For this review, take the finished solid that the model builds, in its own axes (mm). A direction names the side the tool comes from. Round coordinates to 2 decimals unless told otherwise and drop trailing zeros. Write each loop counter-clockwise with the first axis right and the second up, starting at its lowest first coordinate (ties: lowest second). Pieces come first, ordered by that corner, then holes.
from build123d import *

# Parameters (mm, degrees)
SKETCH1_R           = 2.032
BOSS_EXTRUDE1_DEPTH = 2.54
BOSS_EXTRUDE2_DEPTH = 7.62
SKETCH4_R           = 2.032
BOSS_EXTRUDE3_DEPTH = 2.54
CUT_EXTRUDE2_DEPTH  = 6.35
FILLET1_R           = 2.54
FILLET2_R           = 0.635
SKETCH6_R           = 1.95
CUT_EXTRUDE3_DEPTH  = 13.7


with BuildPart() as part:
    # Sketch1 → Boss-Extrude1 (new body)
    with BuildSketch(Plane(origin=(0, 0, 0), x_dir=(0, 0, -1), z_dir=(1, 0, 0))):
        with BuildLine():
            Line((19.05, 0), (0, 0))
            Line((0, 0), (-6.736031019, 0))
            ThreePointArc((-6.736031019, 0), (-5.127948142, 11.168903642), (-12.887784973, 19.361294713))
            Line((-12.887784973, 19.361294713), (-44.861814719, 46.190691279))
            ThreePointArc((-44.861814719, 46.190691279), (-45.74830741, 52.924271785), (-39.11761314, 54.394261314))
            Line((-39.11761314, 54.394261314), (15.875, 22.644261314))
            ThreePointArc((15.875, 22.644261314), (18.199261314, 20.32), (19.05, 17.145))
            Line((19.05, 17.145), (19.05, 0))
        make_face()
        with Locations((3.175, 6.35)):
            Circle(SKETCH1_R, mode=Mode.SUBTRACT)
        with Locations((15.875, 6.35)):
            Circle(SKETCH1_R, mode=Mode.SUBTRACT)
    extrude(amount=BOSS_EXTRUDE1_DEPTH)

    # Sketch1_4 → Boss-Extrude2 (add)
    with BuildSketch(Plane(origin=(0, 0, 0), x_dir=(0, 0, -1), z_dir=(1, 0, 0))):
        with BuildLine():
            Line((-6.736031019, 0), (0, 0))
            Line((0, 0), (0, 12.7))
            Line((0, 12.7), (19.05, 12.7))
            Line((19.05, 12.7), (19.05, 17.145))
            ThreePointArc((19.05, 17.145), (18.199261314, 20.32), (15.875, 22.644261314))
            Line((15.875, 22.644261314), (-39.11761314, 54.394261314))
            ThreePointArc((-39.11761314, 54.394261314), (-45.74830741, 52.924271785), (-44.861814719, 46.190691279))
            Line((-44.861814719, 46.190691279), (-12.887784973, 19.361294713))
            ThreePointArc((-12.887784973, 19.361294713), (-5.127948142, 11.168903642), (-6.736031019, 0))
        make_face()
    extrude(amount=-BOSS_EXTRUDE2_DEPTH)

    # Sketch4 → Boss-Extrude3 (add)
    with BuildSketch(Plane.ZY.offset(7.62)):
        with BuildLine():
            Line((-19.05, 0), (6.736031019, 0))
            ThreePointArc((6.736031019, 0), (5.127948142, 11.168903642), (12.887784973, 19.361294713))
            Line((12.887784973, 19.361294713), (44.861814719, 46.190691279))
            ThreePointArc((44.861814719, 46.190691279), (45.74830741, 52.924271785), (39.11761314, 54.394261314))
            Line((39.11761314, 54.394261314), (-15.875, 22.644261314))
            ThreePointArc((-15.875, 22.644261314), (-18.199261314, 20.32), (-19.05, 17.145))
            Line((-19.05, 17.145), (-19.05, 0))
        make_face()
        with Locations((-3.175, 6.35)):
            Circle(SKETCH4_R, mode=Mode.SUBTRACT)
        with Locations((-15.875, 6.35)):
            Circle(SKETCH4_R, mode=Mode.SUBTRACT)
    extrude(amount=BOSS_EXTRUDE3_DEPTH)

    # Sketch5 → Cut-Extrude2 (cut)
    with BuildSketch(Plane(origin=(2.54, 0, 0), x_dir=(0, 0, -1), z_dir=(1, 0, 0))):
        with BuildLine():
            Line((-19.229074876, 24.682268731), (-13.542236075, 39.628310481))
            Line((-13.542236075, 39.628310481), (-39.11761314, 54.394261314))
            ThreePointArc((-39.11761314, 54.394261314), (-45.74830741, 52.924271785), (-44.861814719, 46.190691279))
            Line((-44.861814719, 46.190691279), (-19.229074876, 24.682268731))
        make_face()
    extrude(amount=-CUT_EXTRUDE2_DEPTH, mode=Mode.SUBTRACT)

    # Fillet1
    fillet1_edges = [part.edges().sort_by_distance(p)[0] for p in [
        (-3.81, 19.361294713, 12.887784973),
        (-3.81, 0, 6.736031019),
        (-0.635, 39.628310481, 13.542236075),
        (-0.635, 24.682268731, 19.229074876),
    ]]
    fillet(fillet1_edges, radius=FILLET1_R)

    # Fillet2
    fillet2_edges = [part.edges().sort_by_distance(p)[0] for p in [
        (1.27, 0, -19.05),
        (-3.81, 12.7, -19.05),
        (-3.81, 0, 0),
        (-8.89, 0, -19.05),
    ]]
    fillet(fillet2_edges, radius=FILLET2_R)

    # Sketch6 → Cut-Extrude3 (cut, through all)
    with BuildSketch(Plane(origin=(2.54, 0, 0), x_dir=(0, 0, -1), z_dir=(1, 0, 0))):
        with Locations((-8.438780502, 24.139537906)):
            Circle(SKETCH6_R)
        with Locations((-0.082541576, 14.180960145)):
            Circle(SKETCH6_R)
    extrude(amount=-CUT_EXTRUDE3_DEPTH, mode=Mode.SUBTRACT)


solid = part.part
(1) Mouldability with a two-part tool opening along Z and no side actions: class faces 1 (the face through (-10.16, 28, 6)), 2 (the face through (1.252, 6.439, -13.845)), 3 (the face through (-8.87, 5.57, -1.3)), 4 (the face through (-0.591, 31.532, 16.623)) as pulls with the +Z half, pulls with the -Z half, needs draft (parallel to the pull), parting line crosses it, or undercut.
Geometry check:
face 1: needs draft
face 2: undercut
face 3: undercut
face 4: pulls with the +Z half
(2) For line 1 along X through (y, z) = (40.5, 21); line 2 along Y through (x, z) = (-9, 24); line 3 along Y through (x, z) = (0.5, -14.5), list the stretches that pass through material, from the lowest coordinate up.
Geometry check:
line 1: x = -10.16 to -3.81
line 2: y = 28.69 to 45.67
line 3: y = 0 to 4.85, 7.85 to 23.44
(3) We need section C-C, the plane z = -4. Give the boundary of the cut face in (x, y), and give its area (3 significant figures).
Geometry check:
outline: (-10.16, 0) - (-7.62, 0) - (-7.62, 4.49) - (-10.16, 4.49) - close; (-10.16, 8.21) - (-7.62, 8.21) - (-7.62, 12.7) - (0, 12.7) - (0, 8.21) - (2.54, 8.21) - (2.54, 29.5) - (-10.16, 29.5) - close; (0, 0) - (2.54, 0) - (2.54, 4.49) - (0, 4.49) - close
area: 259 mm2
(4) We need section B-B, the plane y = 6.35. Give the boundary of the cut face in (x, z), and give its area (3 significant figures).
Geometry check:
outline: (-10.16, -19.05) - (-7.62, -19.05) - (-7.62, -17.91) - (-10.16, -17.91) - close; (-10.16, -13.84) - (-7.62, -13.84) - (-7.62, -5.21) - (-10.16, -5.21) - close; (-10.16, -1.14) - (-7.62, -1.14) - (-7.62, 0) - (0, 0) - (0, -1.14) - (2.54, -1.14) - (2.54, 4.55) - (-10.16, 4.55) - close; (0, -19.05) - (2.54, -19.05) - (2.54, -17.91) - (0, -17.91) - close; (0, -13.84) - (2.54, -13.84) - (2.54, -5.21) - (0, -5.21) - close
area: 113 mm2
(5) For pin 1 Ø9.5 at (y, z) = (38, 21) entering from +X; pin 2 Ø6 at (x, z) = (-3.5, -7.5) entering from -Y; pin 3 Ø2.5 at (x, y) = (-4.5, 4.5) entering from -Z; pin 4 Ø3 at (y, z) = (25.5, 23.5) entering from -X, all flat-tipped, find the tip position at first contact; note any pin that passes through.
Geometry check:
pin 1: stops at x = -3.81
pin 2: stops at y = 12.7
pin 3: stops at z = 0
pin 4: passes through
(6) For faces 5 (the face through (0, 7, -9)), 6 (the face through (-0.679, 24.806, 18.665)), 7 (the face through (-4, 15, -19.05)), 8 (the face through (-3.721, 26.073, 8.693)), 9 (the face through (-0.68, 38.34, 13.05)), list the 3-axis set-ups (+Z, -Z, +X, -X, +Y, -Y) from which the entire face can be reached by the end or side of a thin tool; tool diameter is ignored.
Geometry check:
face 5: -Z, -Y
face 6: +Z, +X
face 7: -Z, +X, -X, +Y, -Y
face 8: +X, -X
face 9: +X, +Y
(7) We need section D-D, the plane z = -13. Give the boundary of the cut face in (x, y).
Geometry check:
outline: (-10.16, 0) - (-7.62, 0) - (-7.62, 12.7) - (0, 12.7) - (0, 0) - (2.54, 0) - (2.54, 24.3) - (-10.16, 24.3) - close
